The listing builds one solid part. Answer for the finished solid, in the listing's coordinates (mm). A direction names the side the tool comes from. Give positions to 0.01 mm unless a question says otherwise; leave off trailing zeros. Order: outer loops, then holes, each group sorted by start corner. A loop starts at its lowest first (then second) coordinate and runs counter-clockwise, first axis right, second up. Notation, with made-up numbers: M 77.5,74 L 129.5,74 A18 cw 129.5,89 Z; hole C -32,52.25 d10. An arc over 180 degrees is marked long. Answer as a JSON object with one key per item and string values. Group by question number.
```python
from build123d import *

# Parameters (mm, degrees)
SKETCH1_R           = 7.5
BOSS_EXTRUDE1_DEPTH = 4
SKETCH2_R           = 11
SKETCH2_R_2         = 7.5
BOSS_EXTRUDE2_DEPTH = 1


with BuildPart() as part:
    # Sketch1 → Boss-Extrude1 (new body, symmetric)
    with BuildSketch(Plane(origin=(0, 0, 0), x_dir=(1, 0, 0), z_dir=(0, 1, 0))):
        Circle(SKETCH1_R)
        Polygon((-2.893968224, -5.0125), (2.893968224, -5.0125), (5.787936449, 0), (2.893968224, 5.0125), (-2.893968224, 5.0125), (-5.787936449, 0), align=None, mode=Mode.SUBTRACT)
    extrude(amount=BOSS_EXTRUDE1_DEPTH, both=True)

    # Sketch2 → Boss-Extrude2 (add)
    with BuildSketch(Plane.XZ.offset(4)):
        Circle(SKETCH2_R)
        Circle(SKETCH2_R_2, mode=Mode.SUBTRACT)
    extrude(amount=-BOSS_EXTRUDE2_DEPTH)


solid = part.part
```
Item 1: Section A-A (x = 0) is taken. Determine the outline of the cut face in (y, z), and give its area (3 significant figures).
Item 2: Consider probe 1 along Y at (x, z) = (-5.75, -7.5); probe 2 along X at (y, z) = (-3.5, -4); probe 3 along Z at (x, y) = (-1.5, -2.5). Determine where each line is inside the solid, lowest interval first. Write a range as from..to.
Item 3: A tool of negligible diameter and unlimited length cuts with its end or side. For faces 4 (the flat face through (7.2, -3, 2.6)), 5 (the flat face through (5, -4, -2)), 6 (the flat face through (-4.32, 0.06, -2.54)), from which of +Z, -Z, +X, -X, +Y, -Y can it reach the whole face along a straight path? Write none if from no direction.
Item 4: Determine the mould class of faces 1 (the flat face through (5, 4, -2)), 2 (the cylindrical face through (-7.493, 0.549, -0.33)), 3 (the flat face through (0, 0, 5.012)) for opening direction X: released by +X, released by -X, zero draft, split by the parting line, or undercut.
Item 5: Flat-ended cylindrical pins translate along their axes: P1, Ø1, axis at x = 3, y = 2, coming from the +Z side; P2, Ø4, axis at y = 2, z = -8.5, coming from the -X side; P3, Ø4, axis at x = -8.5, y = -3, coming from the -Z side. Find the tip coordinate at first contact, or state that the pin passes through.
Item 6: Section B-B (y = 3.25) is taken. Determine the outline of the cut face in (x, z).
Item 7: Section D-D (x = -6.75) is taken. Determine the outline of the cut face in (y, z), and give its area (3 significant figures).
Item 8: Section C-C (z = 2) is taken. Determine the outline of the cut face in (x, y).
Values found:
{
 "1": {"outline": "M -4,-11 L -3,-11 L -3,-7.5 L 4,-7.5 L 4,-5.01 L -4,-5.01 Z; M -4,5.01 L 4,5.01 L 4,7.5 L -3,7.5 L -3,11 L -4,11 Z", "area": "46.8 mm^2"},
 "2": {"probe 1": "y = -4..-3", "probe 2": "x = -10.25..-3.48, 3.48..10.25", "probe 3": "z = -7.35..-5.01, 5.01..7.35"},
 "3": {"face 4": "+Y", "face 5": "+Z, -Z, +X, -X, -Y", "face 6": "+Y, -Y"},
 "4": {"face 1": "zero draft", "face 2": "split by the parting line", "face 3": "undercut"},
 "5": {"P1": "stops at z = 7.07", "P2": "stops at x = -3.74", "P3": "stops at z = -8.87"},
 "6": {"outline": "C 0,0 d15; hole M -5.79,0 L -2.89,-5.01 L 2.89,-5.01 L 5.79,0 L 2.89,5.01 L -2.89,5.01 Z"},
 "7": {"outline": "M -4,-8.69 L -3,-8.69 L -3,-3.27 L 4,-3.27 L 4,3.27 L -3,3.27 L -3,8.69 L -4,8.69 Z", "area": "63.1 mm^2"},
 "8": {"outline": "M -10.82,-4 L -4.63,-4 L -4.63,4 L -7.23,4 L -7.23,-3 L -10.82,-3 Z; M 4.63,-4 L 10.82,-4 L 10.82,-3 L 7.23,-3 L 7.23,4 L 4.63,4 Z"}
}
